Check sheet for the modelled part. Datum: model origin and axes. Units: mm. Give positions to 0.01 mm unless a question says otherwise; leave off trailing zeros. Order: outer loops, then holes, each group sorted by start corner. A loop starts at its lowest first (then second) coordinate and runs counter-clockwise, first axis right, second up. Notation, with made-up numbers: (-33, 81.25) - (12, 81.25) arc R23 ccw to (12, 113.25) - close; hole circle Ø5 at (60.25, -9.75). An arc over 180 degrees is marked (long way). Answer in a Markdown table with one row per item.
from build123d import *

# Parameters (mm, degrees)
BOSS_EXTRUDE2_DEPTH = 1.25
SKETCH5_R           = 1.5
CUT_EXTRUDE3_DEPTH  = 124.258113323


with BuildPart() as part:
    # Sketch2_4 → Boss-Extrude2 (new, symmetric)
    with BuildSketch(Plane(origin=(0, 0, 0), x_dir=(1, 0, 0), z_dir=(0, 1, 0))):
        Polygon((-105, -15), (-105, -55.25), (-75, -55.25), (-75, -60.25), (-45, -60.25), (-45, -55.25), (-15, -55.25), (-15, -60.25), (15, -60.25), (15, -55.25), (45, -55.25), (45, -60.25), (75, -60.25), (75, -55.25), (105, -55.25), (105, -15), (107.5, -15), (107.5, 15), (105, 15), (105, 57.75), (75, 57.75), (75, 60.25), (45, 60.25), (45, 57.75), (15, 57.75), (15, 60.25), (-15, 60.25), (-15, 57.75), (-45, 57.75), (-45, 60.25), (-75, 60.25), (-75, 57.75), (-105, 57.75), (-105, 15), (-107.5, 15), (-107.5, -15), align=None)
    extrude(amount=BOSS_EXTRUDE2_DEPTH, both=True)

    # Sketch5 → Cut-Extrude3 (cut, through all)
    with BuildSketch(Plane(origin=(0, 1.25, 0), x_dir=(1, 0, 0), z_dir=(0, 1, 0))):
        with Locations(Location((98, 50.75, 0), (0, 0, 270))):
            Circle(SKETCH5_R)
        with Locations(Location((-36.37, 50.75, 0), (0, 0, 270))):
            Circle(SKETCH5_R)
        with Locations(Location((-36.37, -25.32, 0), (0, 0, 270))):
            Circle(SKETCH5_R)
        with Locations(Location((98, -25.32, 0), (0, 0, 270))):
            Circle(SKETCH5_R)
        with Locations(Location((53.99, 40.05, 0), (0, 0, 270))):
            Circle(SKETCH5_R)
        with Locations(Location((21.48, 1.57, 0), (0, 0, 270))):
            Circle(SKETCH5_R)
        with Locations(Location((-98, 50.75, 0), (0, 0, 270))):
            Circle(SKETCH5_R)
        with Locations(Location((-57.87, 50.75, 0), (0, 0, 270))):
            Circle(SKETCH5_R)
        with Locations(Location((-98, -25.45, 0), (0, 0, 270))):
            Circle(SKETCH5_R)
        with Locations(Location((-57.87, -25.45, 0), (0, 0, 270))):
            Circle(SKETCH5_R)
        with Locations(Location((-57.87, 9.6, 0), (0, 0, 270))):
            Circle(SKETCH5_R)
        with BuildLine():
            Line((-38, 26), (-38, 24.898979486))
            ThreePointArc((-38, 24.898979486), (-37.777460299, 23.765086067), (-37.142857143, 22.799416849))
            ThreePointArc((-37.142857143, 22.799416849), (-40, 16), (-42.857142857, 22.799416849))
            ThreePointArc((-42.857142857, 22.799416849), (-42.222539701, 23.765086067), (-42, 24.898979486))
            Line((-42, 24.898979486), (-42, 26))
            ThreePointArc((-42, 26), (-40, 28), (-38, 26))
        make_face()
        with BuildLine():
            Line((42, 26), (42, 24.898979486))
            ThreePointArc((42, 24.898979486), (42.222539701, 23.765086067), (42.857142857, 22.799416849))
            ThreePointArc((42.857142857, 22.799416849), (40, 16), (37.142857143, 22.799416849))
            ThreePointArc((37.142857143, 22.799416849), (37.777460299, 23.765086067), (38, 24.898979486))
            Line((38, 24.898979486), (38, 26))
            ThreePointArc((38, 26), (40, 28), (42, 26))
        make_face()
    extrude(amount=-CUT_EXTRUDE3_DEPTH, mode=Mode.SUBTRACT)


solid = part.part
(1) Gauge pin test, flat ends, axial feed: P1, Ø0.8, axis at y = 0.5, z = -29, coming from the +X side; P2, Ø0.8, axis at y = -0.5, z = 57, coming from the -X side; P3, Ø1.2, axis at y = 0, z = -25.5, coming from the -X side; P4, Ø3.5, axis at x = 98, z = -50.75, coming from the +Y side. Record the tip position at first contact, or that the pin passes through.
Geometry says:
| item | result |
|---|---|
| P1 | x = 105 |
| P2 | x = -75 |
| P3 | x = -105 |
| P4 | y = 1.25 |
(2) Mould release check, pull along Z, two halves, no side actions. Record for faces 1 (the cylindrical face through (40, 0, -16)), 2 (the flat face through (-2, -1.25, -1)): pulls with the +Z half, pulls with the -Z half, needs draft (parallel to the pull), parting line crosses it, or undercut.
Geometry says:
| item | result |
|---|---|
| face 1 | undercut |
| face 2 | needs draft |
(3) Cross-section at A-A, the plane z = -20. Record the cut outline in (x, y).
Geometry says:
| item | result |
|---|---|
| outline | (-105, -1.25) - (-44, -1.25) - (-44, 1.25) - (-105, 1.25) - close; (-36, -1.25) - (36, -1.25) - (36, 1.25) - (-36, 1.25) - close; (44, -1.25) - (105, -1.25) - (105, 1.25) - (44, 1.25) - close |
(4) Thickness scan on L1, parallel to X at y = -0.7, z = 25.32; L2, parallel to Z at x = 98, y = 0.05; L3, parallel to Z at x = -98, y = 0. Record the ranges inside material, lowest first.
Geometry says:
| item | result |
|---|---|
| L1 | -105 to -99.49, -96.51 to -59.36, -56.38 to -37.87, -34.87 to 96.5, 99.5 to 105 |
| L2 | -57.75 to -52.25, -49.25 to 23.82, 26.82 to 55.25 |
| L3 | -57.75 to -52.25, -49.25 to 23.95, 26.95 to 55.25 |
(5) Cross-section at B-B, the plane y = -0.65. Give the number of separate pieces and of enclosed holes in the cut face, then the cut area to 3 significant figures.
Geometry says:
| item | result |
|---|---|
| separate pieces | 1 |
| enclosed holes | 13 |
| area | 24,300 mm² |
(6) Cross-section at C-C, the plane x = -21.5. Record the cut outline in (y, z).
Geometry says:
| item | result |
|---|---|
| outline | (-1.25, -57.75) - (1.25, -57.75) - (1.25, 55.25) - (-1.25, 55.25) - close |
(7) Cross-section at D-D, the plane z = -46.5. Record the cut outline in (x, y), then the cut area to 3 significant figures.
Geometry says:
| item | result |
|---|---|
| outline | (-105, -1.25) - (105, -1.25) - (105, 1.25) - (-105, 1.25) - close |
| area | 525 mm² |
